from build123d import *

# Parameters (mm, degrees)
SKETCH_1_W                  = 150
SKETCH_1_H                  = 280
EXTRUDE_1_DEPTH             = 2
SKETCH_4_R                  = 1
CUT_EXTRUDE_1_DEPTH         = 2
PATTERN_LINEAR_1_COUNT      = 2
PATTERN_LINEAR_1_PITCH      = 20
PATTERN_LINEAR_1_COUNT_DIR2 = 2
PATTERN_LINEAR_1_PITCH_DIR2 = 10
MIRROR_2_COPY_1_SKETCH_R    = 1
MIRROR_2_COPY_1_DEPTH       = 2
MIRROR_2_COPY_2_SKETCH_R    = 1
MIRROR_2_COPY_2_DEPTH       = 2
MIRROR_2_COPY_3_SKETCH_R    = 1
MIRROR_2_COPY_3_DEPTH       = 2
CUT_EXTRUDE_2_DEPTH         = 10


with BuildPart() as part:
    # 草图1 → 凸台-拉伸1 (new body)
    with BuildSketch(Plane(origin=(0, 0, 0), x_dir=(1, 0, 0), z_dir=(0, 1, 0))):
        Rectangle(SKETCH_1_W, SKETCH_1_H)
    extrude(amount=EXTRUDE_1_DEPTH)

    # 草图4 → 切除-拉伸1 (cut)
    with BuildSketch(Plane(origin=(0, 2, 0), x_dir=(1, 0, 0), z_dir=(0, 1, 0))):
        with Locations((-55, 132)):
            Circle(SKETCH_4_R)
    cut_extrude_1 = extrude(amount=-CUT_EXTRUDE_1_DEPTH, mode=Mode.SUBTRACT)

    # 阵列(线性)1: Cut-Extrude 1 2 × 2
    with Locations(*[(i * PATTERN_LINEAR_1_PITCH, 0, j * PATTERN_LINEAR_1_PITCH_DIR2) for i in range(PATTERN_LINEAR_1_COUNT) for j in range(PATTERN_LINEAR_1_COUNT_DIR2) if (i, j) != (0, 0)]):
        add(cut_extrude_1, mode=Mode.SUBTRACT)

    # 镜向2: 切除-拉伸1 across plane
    add(cut_extrude_1.mirror(Plane.ZY), mode=Mode.SUBTRACT)

    # 镜向2 copy 1 sketch → 镜向2 copy 1 (cut)
    with BuildSketch(Plane(origin=(0, 2, 10), x_dir=(-1, 0, 0), z_dir=(0, 1, 0))):
        with Locations((-55, -132)):
            Circle(MIRROR_2_COPY_1_SKETCH_R)
    extrude(amount=-MIRROR_2_COPY_1_DEPTH, mode=Mode.SUBTRACT)

    # 镜向2 copy 2 sketch → 镜向2 copy 2 (cut)
    with BuildSketch(Plane(origin=(-20, 2, 0), x_dir=(-1, 0, 0), z_dir=(0, 1, 0))):
        with Locations((-55, -132)):
            Circle(MIRROR_2_COPY_2_SKETCH_R)
    extrude(amount=-MIRROR_2_COPY_2_DEPTH, mode=Mode.SUBTRACT)

    # 镜向2 copy 3 sketch → 镜向2 copy 3 (cut)
    with BuildSketch(Plane(origin=(-20, 2, 10), x_dir=(-1, 0, 0), z_dir=(0, 1, 0))):
        with Locations((-55, -132)):
            Circle(MIRROR_2_COPY_3_SKETCH_R)
    extrude(amount=-MIRROR_2_COPY_3_DEPTH, mode=Mode.SUBTRACT)

    # 草图5 → 切除-拉伸2 (cut)
    with BuildSketch(Plane(origin=(0, 2, 0), x_dir=(1, 0, 0), z_dir=(0, 1, 0))):
        with BuildLine():
            Line((5, 49.5), (5, 29.5))
            ThreePointArc((5, 29.5), (0, 24.5), (-5, 29.5))
            Line((-5, 29.5), (-5, 49.5))
            ThreePointArc((-5, 49.5), (0, 54.5), (5, 49.5))
        make_face()
    extrude(amount=-CUT_EXTRUDE_2_DEPTH, mode=Mode.SUBTRACT)


solid = part.part
Verification items for the finished model (mm, model axes). A direction names the side the tool comes from. Round coordinates to 2 decimals unless told otherwise and drop trailing zeros. Loops run counter-clockwise (first coordinate to the right, second up) from the corner with the lowest first, then second, coordinate; pieces in that order, holes last. Notation, with made-up numbers: (-12, 80.25) - (8, 80.25) arc R23 ccw to (8, 99.25) - close; hole circle Ø6 at (1.5, -21). An arc over 180 degrees is marked (long way). Use a Markdown table: item, result. Add a question column.
1. Section check B-B, the plane x = 0. Record the boundary of the cut face in (y, z), plus the area to 3 significant figures.
2. Gauge pin test, flat end, axial feed: pin 1 (1.8 mm diameter, centred on x = -55, z = -122, fed in from -Y). Record the tip position at first contact, or that the pin passes through.
3. Section check A-A, the plane z = -34. Record the boundary of the cut face in (x, y), plus the area to 3 significant figures.
4. Access from +Z, -Z, +X, -X, +Y, -Y to the whole of each face (thin tool, end or side, straight path). Record for faces 3 (the face through (-1, 0, -2)), 4 (the face through (0.1, 1, -24.5)).
5. Release check for a two-part mould opening along X. For faces 1 (the face through (-1, 2, -2)), 2 (the face through (-0.1, 1, -54.5)) record: released by +X, released by -X, zero draft, split by the parting line, or undercut.
6. Thickness scan on probe 1 along X at (y, z) = (1.3, -132); probe 2 along Z at (x, y) = (55, 1.3); probe 3 along X at (y, z) = (0.25, -29). Record the ranges inside material, lowest first. Write a range as [from, to].
Checks:
| question | item | result |
|---|---|---|
| 1 | outline | (0, -140) - (2, -140) - (2, -54.5) - (0, -54.5) - close; (0, -24.5) - (2, -24.5) - (2, 140) - (0, 140) - close |
| 1 | area | 500 mm^2 |
| 2 | pin 1 | passes through |
| 3 | outline | (-75, 0) - (-5, 0) - (-5, 2) - (-75, 2) - close; (5, 0) - (75, 0) - (75, 2) - (5, 2) - close |
| 3 | area | 280 mm^2 |
| 4 | face 3 | +Z, -Z, +X, -X, -Y |
| 4 | face 4 | +Y, -Y |
| 5 | face 1 | zero draft |
| 5 | face 2 | undercut |
| 6 | probe 1 | x = [-75, -56], [-54, -36], [-34, 34], [36, 54], [56, 75] |
| 6 | probe 2 | z = [-140, -133], [-131, -123], [-121, 140] |
| 6 | probe 3 | x = [-75, -4.97], [4.97, 75] |
